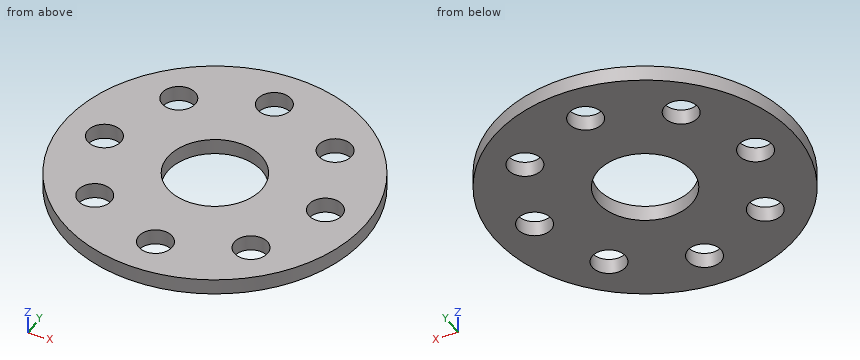
```python
from build123d import *

# Parameters (mm, degrees)
SKETCH1_R            = 24
SKETCH1_R_2          = 7.5
BOSS_EXTRUDE1_DEPTH  = 1.25
M5_CLEARANCE_HOLE1_D = 5.3


with BuildPart() as part:
    # Sketch1 → Boss-Extrude1 (new, symmetric)
    with BuildSketch(Plane.XY):
        Circle(SKETCH1_R)
        Circle(SKETCH1_R_2, mode=Mode.SUBTRACT)
    extrude(amount=BOSS_EXTRUDE1_DEPTH, both=True)

    # M5 Clearance Hole1 (through all)
    with Locations(Plane.XY.offset(1.25)):
        with Locations((0, -17.5), (-12.374368671, -12.374368671), (-17.5, 0), (-12.374368671, 12.374368671), (0, 17.5), (12.374368671, 12.374368671), (17.5, 0), (12.374368671, -12.374368671)):
            Hole(M5_CLEARANCE_HOLE1_D / 2)


solid = part.part
```
Geometry check sheet. Reference: the model listing, model coordinates, mm. Coordinates: 2 decimals unless noted, no trailing zeros. Order: outer loops, then holes, each group sorted by start corner. A loop starts at its lowest first (then second) coordinate and runs counter-clockwise, first axis right, second up. Notation, with made-up numbers: (58.5, 45) - (105.5, 45) arc R23 cw to (105.5, 78) - close; hole circle Ø7 at (27, 70). An arc over 180 degrees is marked (long way). Use one line per item in the form item = value.
1. Scan lines: line 1 (Y direction, x = 0, z = 0.55); line 2 (Y direction, x = -13, z = -1.1). Record each from-to range of solid material in increasing order.
Here are the results:
line_1 = -24 to -20.15, -14.85 to -7.5, 7.5 to 14.85, 20.15 to 24
line_2 = -20.17 to -14.95, -9.8 to 9.8, 14.95 to 20.17
2. Section check A-A (y = 0). Record the boundary of the cut face in (x, z), then the cut area to 3 significant figures.
Here are the results:
outline = (-24, -1.25) - (-20.15, -1.25) - (-20.15, 1.25) - (-24, 1.25) - close; (-14.85, -1.25) - (-7.5, -1.25) - (-7.5, 1.25) - (-14.85, 1.25) - close; (7.5, -1.25) - (14.85, -1.25) - (14.85, 1.25) - (7.5, 1.25) - close; (20.15, -1.25) - (24, -1.25) - (24, 1.25) - (20.15, 1.25) - close
area = 56.0 mm²
3. Section check C-C (x = 17.5). Record the boundary of the cut face in (y, z).
Here are the results:
outline = (-16.42, -1.25) - (-2.65, -1.25) - (-2.65, 1.25) - (-16.42, 1.25) - close; (2.65, -1.25) - (16.42, -1.25) - (16.42, 1.25) - (2.65, 1.25) - close
4. Gauge pin test, flat ends, axial feed: pin 1 (6 mm diameter, centred on x = -17.5, y = 0, fed in from -Z); pin 2 (3 mm diameter, centred on x = 17.5, y = 0, fed in from +Z). Record the tip position at first contact, or that the pin passes through.
Here are the results:
pin_1 = -1.25
pin_2 = through
